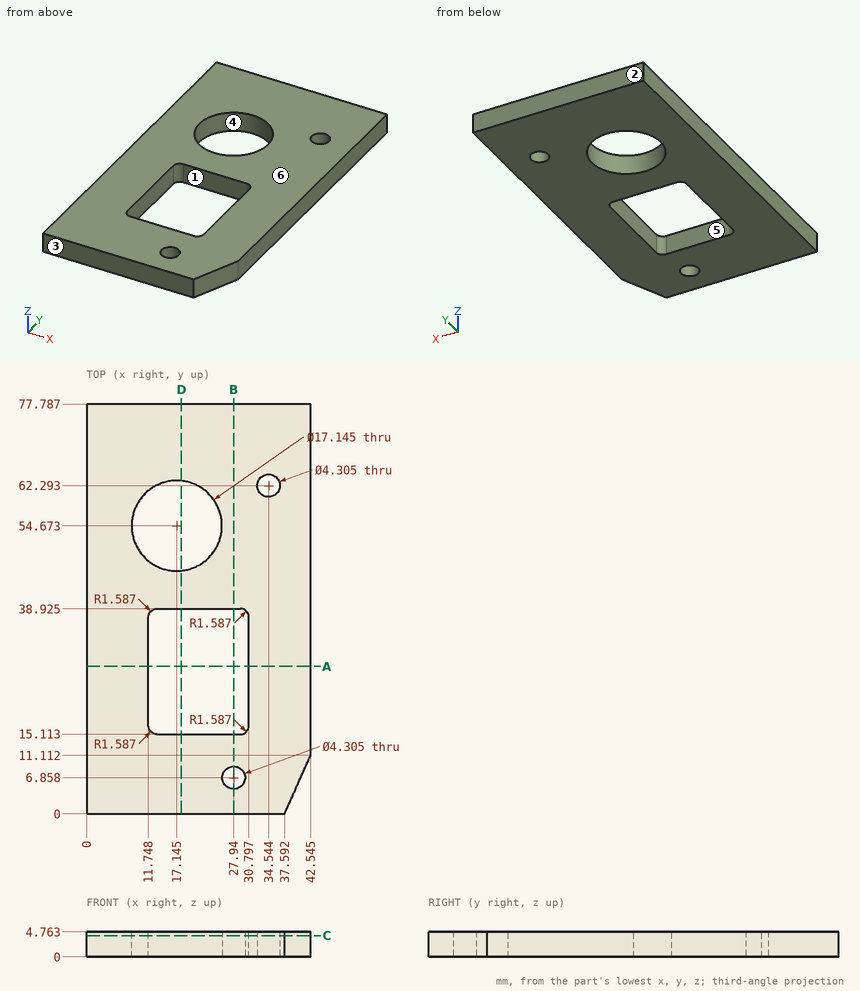
Geometry: see drawing. Coordinates: mm, zero at the bounding-box minimum. A direction names the side the tool comes from. Round coordinates to 2 decimals unless told otherwise and drop trailing zeros. Write each loop counter-clockwise with the first axis right and the second up, starting at its lowest first coordinate (ties: lowest second). Pieces come first, ordered by that corner, then holes.
Item 1: Set-up query: the marked faces 5 and 6. Return all of +Z, -Z, +X, -X, +Y, -Y with unobstructed straight access to the full face (end or side cutting, diameter ignored); none if empty.
Item 2: Section query B-B (x = 27.94). Return loops of the section in (y, z) (1 decimal).
Item 3: Pin query (flat end, axial travel): P1, Ø15.5, axis at x = 17.14, y = 54.67, coming from the +Z side. Return the tip coordinate at first contact, or that it passes through.
Item 4: Section query D-D (x = 18). Return loops of the section in (y, z) (1 decimal).
Item 5: Section query A-A (y = 28). Return loops of the section in (x, z) (1 decimal).
Item 6: Mould query, pull axis Y, two halves, no side actions, for the marked faces 1, 2, 3 and 4. Classes: +Y half, -Y half, draft (parallel to the pull), parting line (faces both ways), or undercut.
Item 7: Section query C-C (z = 4.05). Return loops of the section in (x, y) (1 decimal).
Item 8: Material intervals for L1, parallel to Y at x = 17, z = 2.5 (1 decimal); L2, parallel to Y at x = 27.94, z = 1.05 (1 decimal); L3, parallel to X at y = 20, z = 1.1 (1 decimal), sorted ascending.
Completed:
1. face 5: +Z, -Z
1. face 6: +Z, +X, -X, +Y, -Y
2. outline: (0, 0) - (4.7, 0) - (4.7, 4.8) - (0, 4.8) - close; (9, 0) - (15.1, 0) - (15.1, 4.8) - (9, 4.8) - close; (38.9, 0) - (77.8, 0) - (77.8, 4.8) - (38.9, 4.8) - close
3. P1: passes through
4. outline: (0, 0) - (15.1, 0) - (15.1, 4.8) - (0, 4.8) - close; (38.9, 0) - (46.1, 0) - (46.1, 4.8) - (38.9, 4.8) - close; (63.2, 0) - (77.8, 0) - (77.8, 4.8) - (63.2, 4.8) - close
5. outline: (0, 0) - (11.7, 0) - (11.7, 4.8) - (0, 4.8) - close; (30.8, 0) - (42.5, 0) - (42.5, 4.8) - (30.8, 4.8) - close
6. face 1: undercut
6. face 2: +Y half
6. face 3: -Y half
6. face 4: undercut
7. outline: (0, 0) - (37.6, 0) - (42.5, 11.1) - (42.5, 77.8) - (0, 77.8) - close; hole circle Ø17.1 at (17.1, 54.7); hole (11.7, 16.7) arc R1.6 ccw to (13.3, 15.1) - (29.2, 15.1) arc R1.6 ccw to (30.8, 16.7) - (30.8, 37.3) arc R1.6 ccw to (29.2, 38.9) - (13.3, 38.9) arc R1.6 ccw to (11.7, 37.3) - close; hole circle Ø4.3 at (27.9, 6.9); hole circle Ø4.3 at (34.5, 62.3)
8. L1: y = 0 to 15.1, 38.9 to 46.1, 63.2 to 77.8
8. L2: y = 0 to 4.7, 9 to 15.1, 38.9 to 77.8
8. L3: x = 0 to 11.7, 30.8 to 42.5
